Study the drawing (mm; zero at the part's minimum x, y, z) and answer. A direction names the side the tool comes from. Round coordinates to 2 decimals unless told otherwise and drop trailing zeros. Write each loop counter-clockwise with the first axis right and the second up, starting at its lowest first coordinate (ties: lowest second). Pieces come first, ordered by that corner, then holes. Notation, with made-up numbers: (-16.75, 74) - (35.25, 74) arc R24 cw to (35.25, 113) - close; hole circle Ø6 at (-13.5, 61.5). An arc over 180 degrees is marked (long way). Use one line per item in the form item = value. Start each with the question number.
1) The part is cut by section D-D, the plane x = 27.5. Give the vertices of the cut face in (y, z), plus the area to 3 significant figures.
2) For the marked faces 1 and 2, determine the directions among +Z, -Z, +X, -X, +Y, -Y from which every point of the face is accessible in a straight line to the end or side of a thin tool.
3) The part is cut by section B-B, the plane y = 5.5. Give the vertices of the cut face in (x, z).
4) The part is cut by section A-A, the plane y = 12. Give the vertices of the cut face in (x, z).
5) The part is cut by section C-C, the plane z = 1.5. Give the vertices of the cut face in (x, y).
6) For a pull along X with two mould halves and no side action, classify the marked faces 3, 4, 5 and 6 as released by +X, released by -X, zero draft, split by the parting line, or undercut.
7) Consider line 1 along X through (y, z) = (35, 12.75); line 2 along Y through (x, z) = (22.5, 4.5); line 3 along Y through (x, z) = (54.9, 10). Determine where each line is inside the solid, lowest interval first. Write a range as from..to.
8) Each of these flat-tipped pins is pushed along its axis until it touches: pin 1 (2 mm diameter, centred on y = 5.5, z = 10, fed in from +X); pin 2 (5 mm diameter, centred on x = 45.5, z = 6, fed in from -Y). Where does it stop, or does it pass through?
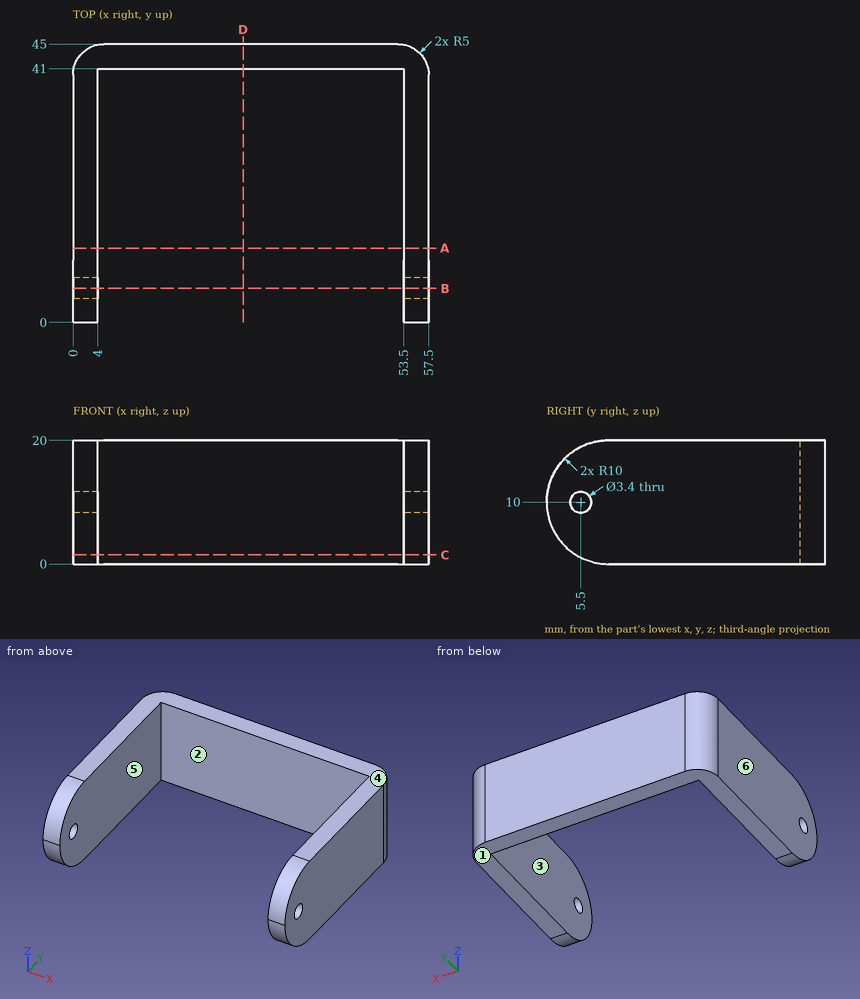
Geometry results:
q1.outline = (41, 0) - (45, 0) - (45, 20) - (41, 20) - close
q1.area = 80.0 mm2
q2.face_1 = -Z, +X, -X, +Y, -Y
q2.face_2 = +Z, -Z, -Y
q3.outline = (0, 1.07) - (4, 1.07) - (4, 8.3) - (0, 8.3) - close; (0, 11.7) - (4, 11.7) - (4, 18.93) - (0, 18.93) - close; (53.5, 1.07) - (57.5, 1.07) - (57.5, 8.3) - (53.5, 8.3) - close; (53.5, 11.7) - (57.5, 11.7) - (57.5, 18.93) - (53.5, 18.93) - close
q4.outline = (0, 0) - (4, 0) - (4, 20) - (0, 20) - close; (53.5, 0) - (57.5, 0) - (57.5, 20) - (53.5, 20) - close
q5.outline = (0, 4.73) - (4, 4.73) - (4, 41) - (53.5, 41) - (53.5, 4.73) - (57.5, 4.73) - (57.5, 40) arc R5 ccw to (52.5, 45) - (5, 45) arc R5 ccw to (0, 40) - close
q6.face_3 = undercut
q6.face_4 = zero draft
q6.face_5 = undercut
q6.face_6 = released by -X
q7.line_1 = 0..4, 53.5..57.5
q7.line_2 = 41..45
q7.line_3 = 0..3.8, 7.2..44.39
q8.pin_1 = through
q8.pin_2 = 41
